from build123d import *

# Parameters (mm, degrees)
BOSS_EXTRUDE1_DEPTH = 7.5
SKETCH2_R           = 2
CUT_EXTRUDE1_DEPTH  = 15
SKETCH3_R           = 11
CUT_EXTRUDE3_DEPTH  = 35
SKETCH4_R           = 6
CUT_EXTRUDE4_DEPTH  = 19.95
CUT_EXTRUDE5_DEPTH  = 6.2
SKETCH7_R           = 20
CUT_EXTRUDE6_DEPTH  = 2.6


with BuildPart() as part:
    # Sketch1 → Boss-Extrude1 (new, symmetric)
    with BuildSketch(Plane.XY):
        with BuildLine():
            Line((-59, 30), (59, 30))
            ThreePointArc((59, 30), (60.414213562, 29.414213562), (61, 28))
            Line((61, 28), (61, -28))
            ThreePointArc((61, -28), (60.414213562, -29.414213562), (59, -30))
            Line((59, -30), (-59, -30))
            ThreePointArc((-59, -30), (-60.414213562, -29.414213562), (-61, -28))
            Line((-61, -28), (-61, 28))
            ThreePointArc((-61, 28), (-60.414213562, 29.414213562), (-59, 30))
        make_face()
    extrude(amount=BOSS_EXTRUDE1_DEPTH, both=True)

    # Sketch2 → Cut-Extrude1 (cut)
    with BuildSketch(Plane(origin=(61, 0, 0), x_dir=(0, 0, -1), z_dir=(1, 0, 0))):
        with Locations(Location((0, 24, 0), (0, 0, 90))):
            Circle(SKETCH2_R)
        with Locations(Location((0, -24, 0), (0, 0, 270))):
            Circle(SKETCH2_R)
    extrude(amount=-CUT_EXTRUDE1_DEPTH, mode=Mode.SUBTRACT)

    # Sketch3 → Cut-Extrude3 (cut)
    with BuildSketch(Plane(origin=(0, 0, -7.5), x_dir=(-1, 0, 0), z_dir=(0, 0, -1))):
        with Locations((36, -0.850791996)):
            Circle(SKETCH3_R)
    extrude(amount=-CUT_EXTRUDE3_DEPTH, mode=Mode.SUBTRACT)

    # Sketch4 → Cut-Extrude4 (cut)
    with BuildSketch(Plane.XY.offset(7.5)):
        with Locations((32.5, 0)):
            Circle(SKETCH4_R)
    extrude(amount=-CUT_EXTRUDE4_DEPTH, mode=Mode.SUBTRACT)

    # Sketch6 → Cut-Extrude5 (cut)
    with BuildSketch(Plane(origin=(0, 0, -7.5), x_dir=(-1, 0, 0), z_dir=(0, 0, -1))):
        Polygon((49.1, 15.249208004), (52.1, 12.249208004), (52.1, -13.950791996), (49.1, -16.950791996), (22.9, -16.950791996), (19.9, -13.950791996), (19.9, 12.249208004), (22.9, 15.249208004), align=None)
    extrude(amount=-CUT_EXTRUDE5_DEPTH, mode=Mode.SUBTRACT)

    # Sketch7 → Cut-Extrude6 (cut)
    with BuildSketch(Plane.XY.offset(7.5)):
        with Locations((32.5, 0)):
            Circle(SKETCH7_R)
    extrude(amount=-CUT_EXTRUDE6_DEPTH, mode=Mode.SUBTRACT)


solid = part.part
CAD build for the part. Positions are in the model's coordinates, mm. A direction names the side the tool comes from. Round coordinates to 2 decimals unless told otherwise and drop trailing zeros. Order: outer loops, then holes, each group sorted by start corner. A loop starts at its lowest first (then second) coordinate and runs counter-clockwise, first axis right, second up. Notation, with made-up numbers: (65.25, -34) -> (115.25, -34) arc R9 cw to (115.25, -19) -> close; hole circle Ø4 at (40.25, 12.25). An arc over 180 degrees is marked (long way). Write item = value, one per line. Start each with the question number.
(1) Cut at A-A, the plane x = 32.5. List the corners of the cut face in (y, z), then the cut area to 3 significant figures.
(2) Cut at B-B, the plane z = -6. List the corners of the cut face in (x, y).
(3) Probe line 1 (Y direction, x = -36, z = 4.75); line 2 (Y direction, x = -30, z = -1.5); line 3 (X direction, y = -2.5, z = -4.5). List the from-to ranges inside material, lowest first. Write a range as [from, to].
(4) Pin check, flat tip, straight feed: P1, Ø3.5, axis at y = 24, z = 0, coming from the +X side. Stop position of the tip, or through.
(5) Which spindle directions (+Z, -Z, +X, -X, +Y, -Y) get a long thin tool onto all of the face, cutting with end or side? Do faces 5 (the flat face through (37, 5, 4.9)), 6 (the flat face through (-19.9, -1, -4)), 7 (the cylindrical face through (53.6, -22.4, 1.2)). Say none if no direction does.
(6) Cut at C-C, the plane y = 24. List the corners of the cut face in (x, z).
(7) Pull direction Z, two halves, no side cores. Call faces 1 (the flat face through (-47, -4, -1.3)), 2 (the cylindrical face through (53.6, 22.4, -1.2)), 3 (the flat face through (46, 24, 0)), 4 (the flat face through (-36, 15.249, -4)): released by +Z, released by -Z, zero draft, split by the parting line, or undercut.
(8) Cut at D-D, the plane x = -36. List the corners of the cut face in (y, z), then the cut area to 3 significant figures.
Model answer:
q1.outline = (-30, -7.5) -> (-6, -7.5) -> (-6, 4.9) -> (-20, 4.9) -> (-20, 7.5) -> (-30, 7.5) -> close; (6, -7.5) -> (30, -7.5) -> (30, 7.5) -> (20, 7.5) -> (20, 4.9) -> (6, 4.9) -> close
q1.area = 647 mm2
q2.outline = (-61, -28) arc R2 ccw to (-59, -30) -> (59, -30) arc R2 ccw to (61, -28) -> (61, 28) arc R2 ccw to (59, 30) -> (-59, 30) arc R2 ccw to (-61, 28) -> close; hole (-52.1, -13.95) -> (-49.1, -16.95) -> (-22.9, -16.95) -> (-19.9, -13.95) -> (-19.9, 12.25) -> (-22.9, 15.25) -> (-49.1, 15.25) -> (-52.1, 12.25) -> close; hole circle Ø12 at (32.5, 0)
q3.line_1 = [-30, -11.85], [10.15, 30]
q3.line_2 = [-30, -16.95], [15.25, 30]
q3.line_3 = [-61, -52.1], [-19.9, 27.05], [37.95, 61]
q4.P1 = 46
q5.face_5 = +Z
q5.face_6 = -Z
q5.face_7 = +X
q6.outline = (-61, -7.5) -> (61, -7.5) -> (61, -2) -> (46, -2) -> (46, 2) -> (61, 2) -> (61, 7.5) -> (-61, 7.5) -> close
q7.face_1 = released by -Z
q7.face_2 = undercut
q7.face_3 = undercut
q7.face_4 = zero draft
q8.outline = (-30, -7.5) -> (-16.95, -7.5) -> (-16.95, -1.3) -> (-11.85, -1.3) -> (-11.85, 7.5) -> (-30, 7.5) -> close; (10.15, -1.3) -> (15.25, -1.3) -> (15.25, -7.5) -> (30, -7.5) -> (30, 7.5) -> (10.15, 7.5) -> close
q8.area = 507 mm2
